Could you check a few things on this drawing? It's one solid part, dimensions in mm from its lowest x, y, z. A direction names the side the tool comes from. Give positions to 0.01 mm unless a question says otherwise; leave off trailing zeros. Order: outer loops, then holes, each group sorted by start corner. A loop starts at its lowest first (then second) coordinate and runs counter-clockwise, first axis right, second up. Notation, with made-up numbers: (-29.75, 55) - (-5.75, 55) arc R11 cw to (-5.75, 74) - close; hole circle Ø10 at (-38, -14). An arc over 180 degrees is marked (long way). Answer as CSV lines item,"result".
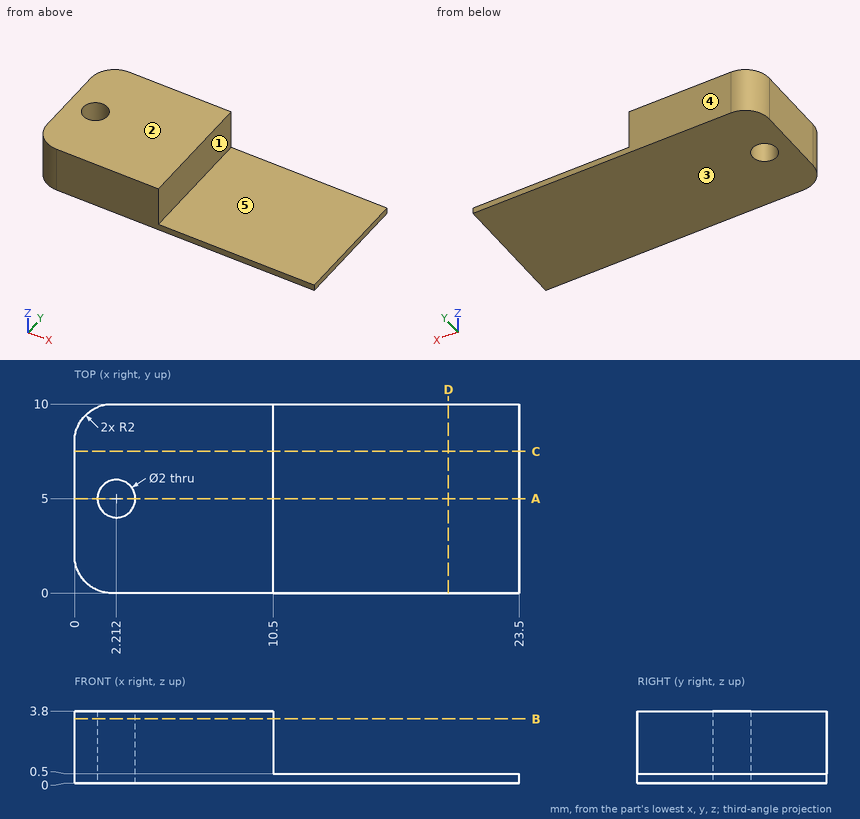
1) I want a section at C-C on y = 7.5. Write out the boundary of the cut face in (x, z).
Answer block:
outline,"(0, 0) - (23.5, 0) - (23.5, 0.5) - (10.5, 0.5) - (10.5, 3.8) - (0, 3.8) - close"
2) I want a section at B-B on z = 3.4. Write out the boundary of the cut face in (x, y), plus the area to 3 significant figures.
Answer block:
outline,"(0, 2) arc R2 ccw to (2, 0) - (10.5, 0) - (10.5, 10) - (2, 10) arc R2 ccw to (0, 8) - close; hole circle Ø2 at (2.21, 5)"
area,"100 mm2"
3) I need wall thicknesses on line 1 along Z through (x, y) = (14, 8); line 2 along X through (y, z) = (7, 3.05); line 3 along Y through (x, z) = (2, 3.2). Which ranges of each line are inside material? Lowest first, please. Write a range as [from, to].
Answer block:
line 1,"[0, 0.5]"
line 2,"[0, 10.5]"
line 3,"[0, 4.02], [5.98, 10]"
4) I want a section at A-A on y = 5. Write out the boundary of the cut face in (x, z).
Answer block:
outline,"(0, 0) - (1.21, 0) - (1.21, 3.8) - (0, 3.8) - close; (3.21, 0) - (23.5, 0) - (23.5, 0.5) - (10.5, 0.5) - (10.5, 3.8) - (3.21, 3.8) - close"
5) Which directions (+Z, -Z, +X, -X, +Y, -Y) give clear straight access to the entire face, cutting with the end or side of a thin tool? Please do the marked faces 4 and 5.
Answer block:
face 4,"+Z, -Z, +X, -X, +Y"
face 5,"+Z, +X, +Y, -Y"
6) I'm going to push a flat-ended pin straight in: P1, Ø2, axis at x = 14.5, y = 8, coming from the +Z side. Where does the tip first touch, or does it pass through?
Answer block:
P1,"z = 0.5"
7) I want a section at D-D on x = 19.75. Write out the boundary of the cut face in (y, z).
Answer block:
outline,"(0, 0) - (10, 0) - (10, 0.5) - (0, 0.5) - close"
8) If we mould it in two halves opening along Z, with no side actions, what happens to the marked faces 1, 2 and 3? For each: +Z half, -Z half, draft (parallel to the pull), parting line (faces both ways), or undercut.
Answer block:
face 1,"draft"
face 2,"+Z half"
face 3,"-Z half"
